For this review, take the finished solid that the model builds, in its own axes (mm). Face numbers are marked on the shaded views. A direction names the side the tool comes from. Coordinates: 2 decimals unless noted, no trailing zeros. Loops run counter-clockwise (first coordinate to the right, second up) from the corner with the lowest first, then second, coordinate; pieces in that order, holes last. Notation, with made-up numbers: (18, -1.75) - (69, -1.75) arc R29 cw to (69, 37.25) - close; hole circle Ø3 at (-15.75, 47.25). An arc over 180 degrees is marked (long way). Use one line per item in the form item = value. Start each with the question number.
1. Add section B-B on y = -20.5. Give the boundary of the cut face in (x, z), and give its area (3 significant figures).
2. Add section C-C on x = -2. Give the boundary of the cut face in (y, z), and give its area (3 significant figures).
3. Machinability: for the marked faces 1, 2 and 3, which of the approach directions +Z, -Z, +X, -X, +Y, -Y give a long, thin tool a straight path to every point of the face, cutting with its end or side? Answer none if there is none.
4. Add section A-A on z = 0. Give the boundary of the cut face in (x, y), and give its area (3 significant figures).
5. To check wall thickness, follow probe 1 along Y at (x, z) = (-19, -1.75); probe 2 along Z at (x, y) = (-5, 1.5); probe 3 along Y at (x, z) = (5, 1). State the ranges of each line that lie inside material, in increasing order.
6. For pin 1 Ø4 at (x, y) = (-0.5, -11.5) entering from +Z; pin 2 Ø1.5 at (x, z) = (-4.5, -2.5) entering from -Y; pin 3 Ø4 at (x, y) = (-18.5, -1.5) entering from -Z, all flat-tipped, find the tip position at first contact; note any pin that passes through.
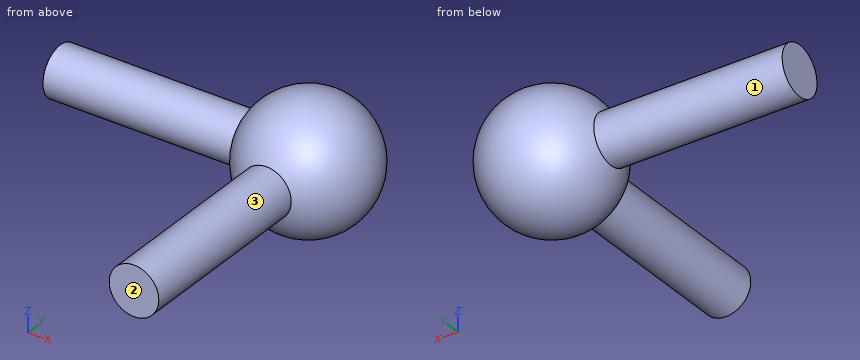
```python
from build123d import *

# Parameters (mm, degrees)
SKETCH_3_R      = 2.5
EXTRUDE_2_DEPTH = 25
SKETCH_2_R      = 2.5
EXTRUDE_1_DEPTH = 25


with BuildPart() as part:
    # 스케치1 → 회전1 (revolve)
    with BuildSketch(Plane.XY):
        with BuildLine():
            Line((0, -6.5), (0, 6.5))
            ThreePointArc((0, 6.5), (-6.5, 0), (0, -6.5))
        make_face()
    revolve(axis=Axis((0, 7.642806544, 0), (0, -1, 0)))

    # 스케치3 → 보스-돌출2 (add)
    with BuildSketch(Plane(origin=(0, 0, 0), x_dir=(0, 0, -1), z_dir=(1, 0, 0))):
        Circle(SKETCH_3_R)
    extrude(amount=-EXTRUDE_2_DEPTH)

    # 스케치2 → 보스-돌출1 (add)
    with BuildSketch(Plane(origin=(0, 0, 0), x_dir=(1, 0, 0), z_dir=(0, 1, 0))):
        Circle(SKETCH_2_R)
    extrude(amount=-EXTRUDE_1_DEPTH)


solid = part.part
```
Conclusion:
q1.outline = circle Ø5 at (0, 0)
q1.area = 19.6 mm^2
q2.outline = (-25, -1.5) - (-6, -1.5) arc R6.18 ccw (long way) to (-6, 1.5) - (-25, 1.5) - close
q2.area = 177 mm^2
q3.face_1 = -X
q3.face_2 = +Z, -Z, +X, -X, -Y
q3.face_3 = -Y
q4.outline = (-25, -2.5) - (-6, -2.5) arc R6.5 ccw to (-2.5, -6) - (-2.5, -25) - (2.5, -25) - (2.5, -6) arc R6.5 ccw (long way) to (-6, 2.5) - (-25, 2.5) - close
q4.area = 319 mm^2
q5.probe_1 = -1.79 to 1.79
q5.probe_2 = -3.87 to 3.87
q5.probe_3 = -4.03 to 4.03
q6.pin_1 = 2.5
q6.pin_2 = -4.79
q6.pin_3 = -2.5
